Geometry check sheet. Reference: the model listing, model coordinates, mm. Face numbers are marked on the shaded views. A direction names the side the tool comes from. Give positions to 0.01 mm unless a question says otherwise; leave off trailing zeros. Write each loop counter-clockwise with the first axis right and the second up, starting at its lowest first coordinate (ties: lowest second). Pieces come first, ordered by that corner, then holes. Notation, with made-up numbers: (-27, 21.5) - (16, 21.5) arc R24 ccw to (16, 53.5) - close; hole circle Ø2 at (-4, 51). An arc over 180 degrees is marked (long way). Write item = value, one per line. Start each with the question number.
(1) Section check B-B, the plane z = 1. Enter the section's corners in (x, y), plus the area to 3 significant figures.
(2) Depth check by flat-ended pin: pin 1 Ø3.5 at (x, y) = (19.5, -1) entering from +Z; pin 2 Ø3.5 at (y, z) = (-34, 9) entering from -X; pin 3 Ø3 at (y, z) = (6, 4.5) entering from -X. Enter the tip coordinate at first touch or a pass-through.
(3) Section check A-A, the plane x = -20. Enter the section's corners in (y, z), plus the area to 3 significant figures.
(4) Access from +Z, -Z, +X, -X, +Y, -Y to the whole of each face (thin tool, end or side, straight path). Record for the marked faces 1 and 2.
(5) Draft check along X on the marked faces 3, 4 and 5. Enter one of: pulls with the +X half, pulls with the -X half, needs draft (parallel to the pull), parting line crosses it, or undercut.
(6) Thickness scan on L1, parallel to X at y = -3, z = 8; L2, parallel to Y at x = 0, z = 2.7; L3, parallel to Y at x = 3, z = 3.5. Record the ranges inside material, lowest first.
(7) Section check D-D, the plane y = 0. Enter the section's corners in (x, z), plus the area to 3 significant figures.
```python
from build123d import *

# Parameters (mm, degrees)
EXTRUDE1_DEPTH                 = 10
SKETCH2_R                      = 15.25
EXTRUDE2_DEPTH                 = 11
F_5_3_5_3_DIAMETER_HOLE1_D     = 5.3
F_5_3_5_3_DIAMETER_HOLE1_DEPTH = 15
SKETCH4_R                      = 7
EXTRUDE3_DEPTH                 = 8
SKETCH5_W                      = 3
SKETCH5_H                      = 2.962602834
EXTRUDE4_DEPTH                 = 3
SKETCH6_W                      = 1
SKETCH6_H                      = 2.1
EXTRUDE5_DEPTH                 = 3
SKETCH7_R                      = 0.9
EXTRUDE6_DEPTH                 = 5
EXTRUDE7_DEPTH                 = 2
SKETCH9_R                      = 1.5
EXTRUDE9_DEPTH                 = 11
SKETCH10_R                     = 3.5
EXTRUDE10_DEPTH                = 5


with BuildPart() as part:
    # Sketch1 → Extrude1 (new body)
    with BuildSketch(Plane.XY):
        with BuildLine():
            Line((-0.385076955, -35), (11.614923045, -35))
            Line((11.614923045, -35), (23.167030313, -9.396207025))
            ThreePointArc((23.167030313, -9.396207025), (-4.655667218, 24.562670106), (-18.121718507, -17.222175192))
            Line((-18.121718507, -17.222175192), (-0.385076955, -35))
        make_face()
    extrude(amount=EXTRUDE1_DEPTH)

    # Sketch2 → Extrude2 (cut, through all)
    with BuildSketch(Plane.XY.offset(10)):
        Circle(SKETCH2_R)
    extrude(amount=-EXTRUDE2_DEPTH, mode=Mode.SUBTRACT)

    # Ø5.3 (5.3) Diameter Hole1
    with Locations(Plane(origin=(5.5, -25.2, 10), x_dir=(1, 0, 0), z_dir=(0, 0, 1))):
        with Locations((0, 0)):
            Hole(F_5_3_5_3_DIAMETER_HOLE1_D / 2, depth=F_5_3_5_3_DIAMETER_HOLE1_DEPTH)

    # Sketch4 → Extrude3 (cut)
    with BuildSketch(Plane.XY.offset(10)):
        with Locations((5.5, -25.2)):
            Circle(SKETCH4_R)
    extrude(amount=-EXTRUDE3_DEPTH, mode=Mode.SUBTRACT)

    # Sketch5 → Extrude4 (cut)
    with BuildSketch(Plane.XY.offset(10)):
        with Locations((5.5, -33.518698583)):
            Rectangle(SKETCH5_W, SKETCH5_H)
    extrude(amount=-EXTRUDE4_DEPTH, mode=Mode.SUBTRACT)

    # Sketch6 → Extrude5 (cut, through all)
    with BuildSketch(Plane.XY.offset(2)):
        with Locations((0, -24.741008814)):
            Rectangle(SKETCH6_W, SKETCH6_H)
    extrude(amount=-EXTRUDE5_DEPTH, mode=Mode.SUBTRACT)

    # Sketch7 → Extrude6 (cut)
    with BuildSketch(Plane.XY.offset(10)):
        with Locations((-1.44988107, -20.370788479)):
            Circle(SKETCH7_R)
    extrude(amount=-EXTRUDE6_DEPTH, mode=Mode.SUBTRACT)

    # Sketch8 → Extrude7 (cut)
    with BuildSketch(Plane.XY.offset(10)):
        with BuildLine():
            Line((-3.55371741, -22.509449896), (-1.470560637, -24.558685407))
            Line((-1.470560637, -24.558685407), (2.590549038, -18.833282235))
            Line((2.590549038, -18.833282235), (-0.272375103, -17.611535012))
            ThreePointArc((-0.272375103, -17.611535012), (-3.942252339, -18.701032372), (-3.55371741, -22.509449896))
        make_face()
    extrude(amount=-EXTRUDE7_DEPTH, mode=Mode.SUBTRACT)

    # Sketch9 → Extrude9 (cut, through all)
    with BuildSketch(Plane.XY):
        with Locations((0, 20)):
            Circle(SKETCH9_R)
        with Locations((-20, 0)):
            Circle(SKETCH9_R)
        with Locations((20, 0)):
            Circle(SKETCH9_R)
    extrude(amount=EXTRUDE9_DEPTH, mode=Mode.SUBTRACT)

    # Sketch10 → Extrude10 (cut)
    with BuildSketch(Plane.XY.offset(10)):
        with Locations((-20, 0)):
            Circle(SKETCH10_R)
        with Locations((0, 20)):
            Circle(SKETCH10_R)
        with Locations((20, 0)):
            Circle(SKETCH10_R)
    extrude(amount=-EXTRUDE10_DEPTH, mode=Mode.SUBTRACT)


solid = part.part
```
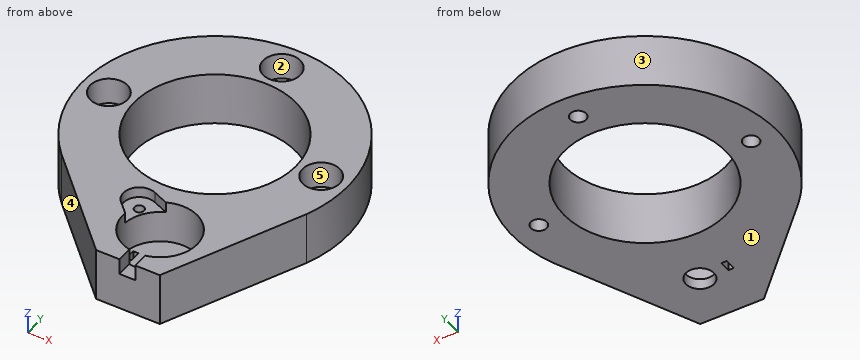
Model answer:
q1.outline = (-18.12, -17.22) - (-0.39, -35) - (11.61, -35) - (23.17, -9.4) arc R25 ccw (long way) to start; hole circle Ø3 at (-20, 0); hole circle Ø30.5 at (0, 0); hole circle Ø3 at (0, 20); hole (-0.5, -25.79) - (0.5, -25.79) - (0.5, -23.69) - (-0.5, -23.69) - close; hole circle Ø5.3 at (5.5, -25.2); hole circle Ø3 at (20, 0)
q1.area = 1,440 mm²
q2.pin_1 = 5
q2.pin_2 = -3.13
q2.pin_3 = -24.59
q3.outline = (-15, 0) - (-1.5, 0) - (-1.5, 5) - (-3.5, 5) - (-3.5, 10) - (-15, 10) - close; (1.5, 0) - (15, 0) - (15, 10) - (3.5, 10) - (3.5, 5) - (1.5, 5) - close
q3.area = 250 mm²
q4.face_1 = -Z, +X, -X, +Y, -Y
q4.face_2 = +Z
q5.face_3 = parting line crosses it
q5.face_4 = pulls with the -X half
q5.face_5 = undercut
q6.L1 = -24.82 to -21.8, -18.2 to -14.95, 14.95 to 18.2, 21.8 to 24.82
q6.L2 = -35 to -29.53, -20.87 to -15.25, 15.25 to 18.5, 21.5 to 25
q6.L3 = -35 to -31.74, -18.66 to -14.95, 14.95 to 24.82
q7.outline = (-25, 0) - (-21.5, 0) - (-21.5, 5) - (-23.5, 5) - (-23.5, 10) - (-25, 10) - close; (-18.5, 0) - (-15.25, 0) - (-15.25, 10) - (-16.5, 10) - (-16.5, 5) - (-18.5, 5) - close; (15.25, 0) - (18.5, 0) - (18.5, 5) - (16.5, 5) - (16.5, 10) - (15.25, 10) - close; (21.5, 0) - (25, 0) - (25, 10) - (23.5, 10) - (23.5, 5) - (21.5, 5) - close
q7.area = 95.0 mm²
